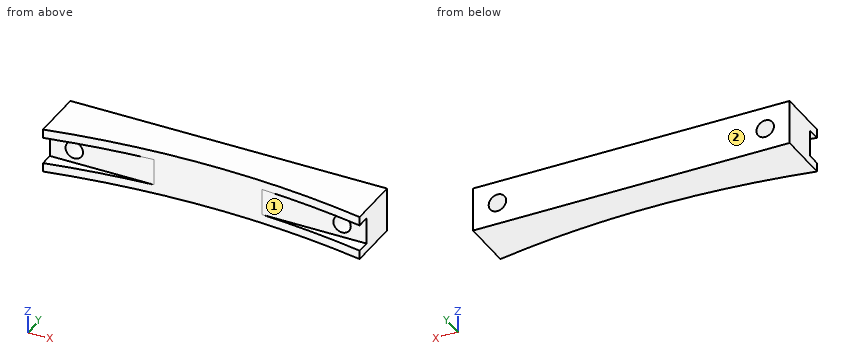
from build123d import *

# Parameters (mm, degrees)
BOSS_EXTRUDE1_DEPTH = 12.7
SKETCH2_R           = 2.5
CUT_EXTRUDE1_DEPTH  = 16.24
SKETCH3_W           = 7.62
SKETCH3_H           = 3.81
CUT_EXTRUDE2_DEPTH  = 91.7700001


with BuildPart() as part:
    # Sketch1 → Boss-Extrude1 (new body)
    with BuildSketch(Plane.XY):
        with BuildLine():
            Line((-45.385, 0), (45.385, 0))
            Line((45.385, 0), (45.385, -15.24))
            ThreePointArc((45.385, -15.24), (0, -10.933442473), (-45.385, -15.24))
            Line((-45.385, -15.24), (-45.385, 0))
        make_face()
    extrude(amount=BOSS_EXTRUDE1_DEPTH)

    # Sketch2 → Cut-Extrude1 (cut, through all)
    with BuildSketch(Plane(origin=(0, 0, 0), x_dir=(1, 0, 0), z_dir=(0, 1, 0))):
        with Locations((-38.385, -6.35)):
            Circle(SKETCH2_R)
        with Locations((38.385, -6.35)):
            Circle(SKETCH2_R)
    extrude(amount=-CUT_EXTRUDE1_DEPTH, mode=Mode.SUBTRACT)

    # Sketch3 → Cut-Extrude2 (cut, through all)
    with BuildSketch(Plane(origin=(45.385, 0, 0), x_dir=(0, 0, -1), z_dir=(1, 0, 0))):
        with Locations((-6.35, -13.335)):
            Rectangle(SKETCH3_W, SKETCH3_H)
    extrude(amount=-CUT_EXTRUDE2_DEPTH, mode=Mode.SUBTRACT)


solid = part.part
For this review, take the finished solid that the model builds, in its own axes (mm). Face numbers are marked on the shaded views. A direction names the side the tool comes from. Coordinates: 2 decimals unless noted, no trailing zeros. Loops run counter-clockwise (first coordinate to the right, second up) from the corner with the lowest first, then second, coordinate; pieces in that order, holes last. Notation, with made-up numbers: (41, 27) - (72, 27) arc R13 cw to (72, 33) - close; hole circle Ø5 at (48, 57). An arc over 180 degrees is marked (long way). Return JSON: item names as keys, results as strings.
Item 1: Insertion check: pin 1 (4 mm diameter, centred on x = 34.5, z = 7.5, fed in from -Y); pin 2 (3 mm diameter, centred on x = 33.5, y = -12.5, fed in from -Z); pin 3 (3 mm diameter, centred on x = -38.385, z = 6.35, fed in from +Y). Each pin has a flat end and moves straight along its axis. Give the tip position at first contact, or say it passes through.
Determined:
{"pin 1": "stops at y = -11.43", "pin 2": "stops at z = 0", "pin 3": "passes through"}
Item 2: For line 1 (X direction, y = -8.25, z = 6.35) (3 decimals); line 2 (Z direction, x = -41, y = -11.75); line 3 (X direction, y = -8, z = 5) (3 decimals), list the stretches that pass through material, from the lowest coordinate up.
Determined:
{"line 1": "x = -45.385 to -40.885, -35.885 to 35.885, 40.885 to 45.385", "line 2": "z = 0 to 2.54, 10.16 to 12.7", "line 3": "x = -45.385 to -40.489, -36.281 to 36.281, 40.489 to 45.385"}
Item 3: For the marked faces 1 and 2, list the 3-axis set-ups (+Z, -Z, +X, -X, +Y, -Y) from which the entire face can be reached by the end or side of a thin tool; tool diameter is ignored.
Determined:
{"face 1": "+X, -X, -Y", "face 2": "+Z, -Z, +X, -X, +Y"}
Item 4: Take a section at B-B (y = -9.25). Give the boundary of the cut face in (x, z) (3 decimals).
Determined:
{"outline": "(-45.385, 0) - (45.385, 0) - (45.385, 12.7) - (-45.385, 12.7) - close; hole circle Ø5 at (-38.385, 6.35); hole circle Ø5 at (38.385, 6.35)"}
Item 5: Take a section at D-D (z = 11.25). Give the boundary of the cut face in (x, y) (3 decimals).
Determined:
{"outline": "(-45.385, -15.24) arc R241.3 cw to (45.385, -15.24) - (45.385, 0) - (-45.385, 0) - close"}
Item 6: Take a section at C-C (x = 25). Give the boundary of the cut face in (y, z).
Determined:
{"outline": "(-12.23, 0) - (0, 0) - (0, 12.7) - (-12.23, 12.7) - (-12.23, 10.16) - (-11.43, 10.16) - (-11.43, 2.54) - (-12.23, 2.54) - close"}
Item 7: Take a section at A-A (z = 6.35). Give the boundary of the cut face in (x, y) (3 decimals), then the cut area to 3 significant figures.
Determined:
{"outline": "(-45.385, -11.43) - (-40.885, -11.43) - (-40.885, 0) - (-45.385, 0) - close; (-35.885, -11.43) - (-15.472, -11.43) arc R241.3 cw to (15.472, -11.43) - (35.885, -11.43) - (35.885, 0) - (-35.885, 0) - close; (40.885, -11.43) - (45.385, -11.43) - (45.385, 0) - (40.885, 0) - close", "area": "913 mm2"}
